Input: dimensioned drawing with shaded views. Units: mm. Origin: part minimum x, y, z. Give positions to 0.01 mm unless a question says otherwise; leave off trailing zeros. Loops run counter-clockwise (first coordinate to the right, second up) from the corner with the lowest first, then second, coordinate; pieces in that order, holes last. Notation, with made-up numbers: M 65,69 L 77,69 A21 ccw 77,75 Z; hole C 78.5,71 d10. An arc over 180 degrees is marked long. Answer in a Markdown table with one row per item.
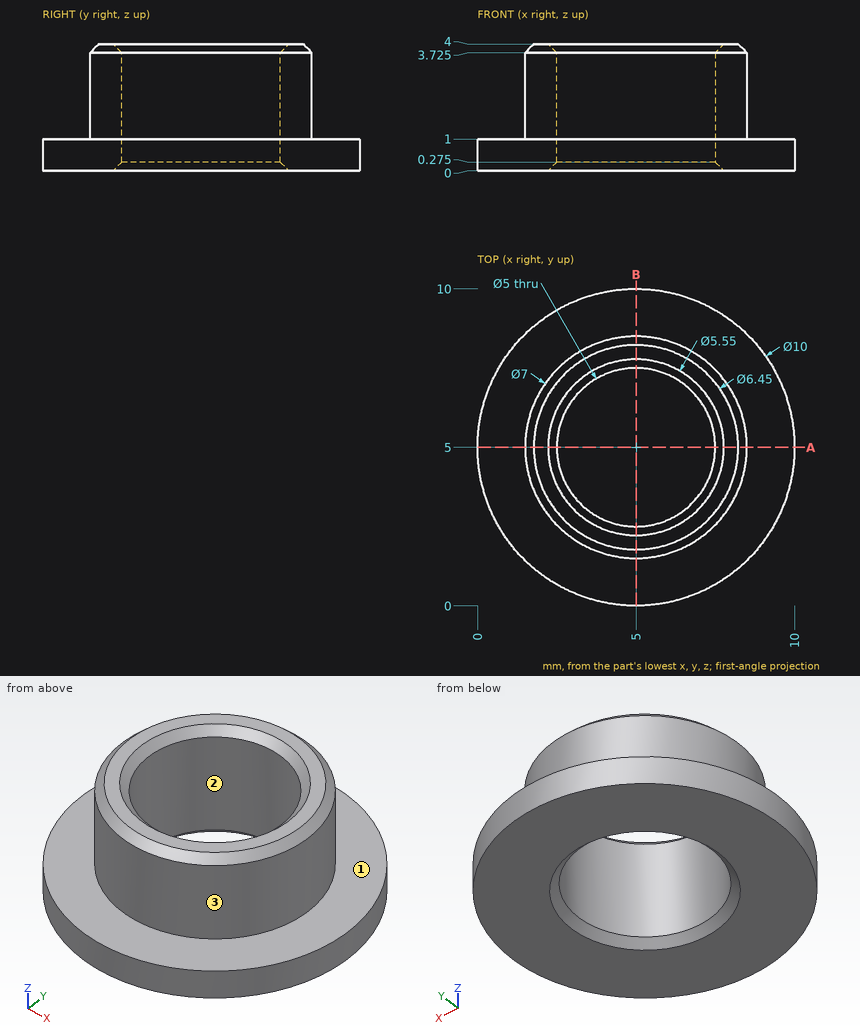
Q1. Ray query, probe 1 along Y at (x, z) = (5, 2.6); probe 2 along Z at (x, y) = (9.25, 2.5); probe 3 along Y at (x, z) = (6, 1.2). Return the intervals inside material, ascending. Write a range as from..to.
Values follow:
| item | result |
|---|---|
| probe 1 | 1.5..2.5, 7.5..8.5 |
| probe 2 | 0..1 |
| probe 3 | 1.65..2.71, 7.29..8.35 |
Q2. Mould query, pull axis Y, two halves, no side actions, for the marked faces 1, 2 and 3. Classes: +Y half, -Y half, draft (parallel to the pull), parting line (faces both ways), or undercut.
Values follow:
| item | result |
|---|---|
| face 1 | draft |
| face 2 | undercut |
| face 3 | parting line |
Q3. Contact query for flat-ended pins moving along their axis: pin 1 Ø2 at (x, z) = (3.5, 1.5) entering from -Y; pin 2 Ø1.5 at (x, y) = (8.5, 6) entering from +Z; pin 3 Ø1.5 at (x, z) = (7, 3.5) entering from +Y. Output: stop coordinate, or through.
Values follow:
| item | result |
|---|---|
| pin 1 | y = 0.04 |
| pin 2 | z = 4 |
| pin 3 | y = 8.27 |
Q4. Section query A-A (y = 5). Output: boundary loops of the cut face in (x, z) (3 decimals).
Values follow:
| item | result |
|---|---|
| outline | M 0,0 L 2.225,0 L 2.5,0.275 L 2.5,3.725 L 2.225,4 L 1.775,4 L 1.5,3.725 L 1.5,1 L 0,1 Z; M 7.5,0.275 L 7.775,0 L 10,0 L 10,1 L 8.5,1 L 8.5,3.725 L 8.225,4 L 7.775,4 L 7.5,3.725 Z |
